```python
from build123d import *
from OCP.BRepFilletAPI import BRepFilletAPI_MakeChamfer

# Parameters (mm, degrees)
SKETCH3_W           = 45.6
SKETCH3_H           = 24.8
BOSS_EXTRUDE1_DEPTH = 29
SKETCH4_W           = 29
SKETCH4_H           = 24.8
BOSS_EXTRUDE2_DEPTH = 1.5
SKETCH6_R           = 12
CUT_EXTRUDE1_DEPTH  = 1.5
BOSS_EXTRUDE3_DEPTH = 1
SKETCH10_W          = 12
SKETCH10_H          = 18.8
BOSS_EXTRUDE5_DEPTH = 1.5
CUT_EXTRUDE2_DEPTH  = 18.8
CUT_EXTRUDE3_DEPTH  = 1.5
SKETCH13_W          = 6
SKETCH13_H          = 20
CUT_EXTRUDE4_DEPTH  = 5
SKETCH14_R          = 0.75
CUT_EXTRUDE5_DEPTH  = 5
SKETCH8_R           = 1
CUT_EXTRUDE6_DEPTH  = 5
CUT_EXTRUDE7_START  = -5
SKETCH15_R          = 0.75
CUT_EXTRUDE7_DEPTH  = 5
SKETCH17_R          = 0.75
CUT_EXTRUDE8_DEPTH  = 5
SKETCH18_R          = 3
BOSS_EXTRUDE6_DEPTH = 3
SKETCH19_R          = 1.5
CUT_EXTRUDE9_DEPTH  = 3
FILLET1_R           = 2
CHAMFER1_SIZE       = 2
CHAMFER2_SIZE       = 1
CHAMFER2_SIZE_2     = 0.577350269
BOSS_EXTRUDE7_START = 3
SKETCH9_R           = 3
SKETCH9_R_2         = 1.25
BOSS_EXTRUDE7_DEPTH = 3


with BuildPart() as part:
    # Sketch3 → Boss-Extrude1 (new body)
    with BuildSketch(Plane(origin=(0, 0, 0), x_dir=(0, 0, -1), z_dir=(1, 0, 0))):
        Rectangle(SKETCH3_W, SKETCH3_H)
    extrude(amount=BOSS_EXTRUDE1_DEPTH)

    # Sketch4 → Boss-Extrude2 (add)
    with BuildSketch(Plane(origin=(29, 0, 0), x_dir=(0, 0, -1), z_dir=(1, 0, 0))):
        with Locations((-8.3, 0)):
            Rectangle(SKETCH4_W, SKETCH4_H)
    boss_extrude2 = extrude(amount=BOSS_EXTRUDE2_DEPTH)

    # Sketch6 → Cut-Extrude1 (cut)
    with BuildSketch(Plane(origin=(29, 0, 0), x_dir=(0, 0, -1), z_dir=(1, 0, 0))):
        with Locations((12.8, 0)):
            Circle(SKETCH6_R)
    cut_extrude1 = extrude(amount=CUT_EXTRUDE1_DEPTH, mode=Mode.SUBTRACT)

    # Sketch7 → Boss-Extrude3 (add)
    with BuildSketch(Plane(origin=(30.5, 0, 0), x_dir=(0, 0, -1), z_dir=(1, 0, 0))):
        with BuildLine():
            Line((-22.8, 7.4), (3.353307457, 7.4))
            ThreePointArc((3.353307457, 7.4), (0.8, 0), (3.353307457, -7.4))
            Line((3.353307457, -7.4), (-22.8, -7.4))
            Line((-22.8, -7.4), (-22.8, 7.4))
        make_face()
    extrude(amount=BOSS_EXTRUDE3_DEPTH)

    # Mirror2: Boss-Extrude2, Cut-Extrude1 across plane
    add(boss_extrude2.mirror(Plane.ZY.offset(-14.5)))
    add(cut_extrude1.mirror(Plane.ZY.offset(-14.5)), mode=Mode.SUBTRACT)

    # Sketch10 → Boss-Extrude5 (add)
    with BuildSketch(Plane.ZY.offset(1.5)):
        with Locations((11.3, 0)):
            Rectangle(SKETCH10_W, SKETCH10_H)
    extrude(amount=BOSS_EXTRUDE5_DEPTH)

    # Sketch11 → Cut-Extrude2 (cut)
    with BuildSketch(Plane.XZ.offset(9.4)):
        Polygon((-3, 7.3), (-1.5, 5.3), (-3, 5.3), align=None)
    extrude(amount=-CUT_EXTRUDE2_DEPTH, mode=Mode.SUBTRACT)

    # Sketch12 → Cut-Extrude3 (cut)
    with BuildSketch(Plane.ZY.offset(1.5)):
        with BuildLine():
            Line((5.3, -10.4), (-0.7, -10.4))
            Line((-0.7, -10.4), (-0.7, -6.479969136))
            Line((-0.7, -6.479969136), (-2.7, -6.479969136))
            ThreePointArc((-2.7, -6.479969136), (-0.8, 0), (-2.7, 6.479969136))
            Line((-2.7, 6.479969136), (-0.7, 6.479969136))
            Line((-0.7, 6.479969136), (-0.7, 9.6))
            Line((-0.7, 9.6), (5.3, 9.6))
            Line((5.3, 9.6), (5.3, -10.4))
        make_face()
    extrude(amount=-CUT_EXTRUDE3_DEPTH, mode=Mode.SUBTRACT)

    # Sketch13 → Cut-Extrude4 (cut)
    with BuildSketch(Plane.ZY):
        with Locations((2.3, -0.4)):
            Rectangle(SKETCH13_W, SKETCH13_H)
    extrude(amount=-CUT_EXTRUDE4_DEPTH, mode=Mode.SUBTRACT)

    # Sketch14 → Cut-Extrude5 (cut)
    with BuildSketch(Plane.ZY.offset(1.5)):
        with Locations((20.8, 10.4)):
            Circle(SKETCH14_R)
        with Locations((20.8, -10.4)):
            Circle(SKETCH14_R)
        with Locations((-3.7, 10.4)):
            Circle(SKETCH14_R)
        with Locations((-3.7, -10.4)):
            Circle(SKETCH14_R)
    extrude(amount=-CUT_EXTRUDE5_DEPTH, mode=Mode.SUBTRACT)

    # Sketch8 → Cut-Extrude6 (cut)
    with BuildSketch(Plane(origin=(30.5, 0, 0), x_dir=(0, 0, -1), z_dir=(1, 0, 0))):
        with Locations((-20.8, 10.4)):
            Circle(SKETCH8_R)
        with Locations((-20.8, -10.4)):
            Circle(SKETCH8_R)
    cut_extrude6 = extrude(amount=-CUT_EXTRUDE6_DEPTH, mode=Mode.SUBTRACT)

    # Sketch15 → Cut-Extrude7 (cut)
    with BuildSketch(Plane(origin=(30.5, 0, 0), x_dir=(0, 0, -1), z_dir=(1, 0, 0)).offset(CUT_EXTRUDE7_START)):
        with Locations(Location((3.7, -10.4, 0), (0, 0, 180))):
            Circle(SKETCH15_R)
        with Locations(Location((3.7, 10.4, 0), (0, 0, 180))):
            Circle(SKETCH15_R)
    extrude(amount=CUT_EXTRUDE7_DEPTH, mode=Mode.SUBTRACT)

    # Sketch17 → Cut-Extrude8 (cut)
    with BuildSketch(Plane(origin=(30.5, 0, 0), x_dir=(0, 0, -1), z_dir=(1, 0, 0))):
        with Locations((-16.8, 10.4)):
            Circle(SKETCH17_R)
        with Locations((-16.8, -10.4)):
            Circle(SKETCH17_R)
    extrude(amount=-CUT_EXTRUDE8_DEPTH, mode=Mode.SUBTRACT)

    # Mirror3: Cut-Extrude6 across plane
    add(cut_extrude6.mirror(Plane.XY), mode=Mode.SUBTRACT)

    # Sketch18 → Boss-Extrude6 (add)
    with BuildSketch(Plane(origin=(29, 0, 0), x_dir=(0, 0, -1), z_dir=(1, 0, 0))):
        with Locations(Location((12.8, 0, 0), (0, 0, 180))):
            Circle(SKETCH18_R)
    extrude(amount=BOSS_EXTRUDE6_DEPTH)

    # Sketch19 → Cut-Extrude9 (cut)
    with BuildSketch(Plane(origin=(32, 0, 0), x_dir=(0, 0, -1), z_dir=(1, 0, 0))):
        with Locations((12.8, 0)):
            Circle(SKETCH19_R)
    extrude(amount=-CUT_EXTRUDE9_DEPTH, mode=Mode.SUBTRACT)

    # Fillet1
    fillet1_edges = [part.edges().sort_by_distance(p)[0] for p in [
        (14.5, -12.4, 22.8),
        (14.5, 12.4, 22.8),
    ]]
    fillet(fillet1_edges, radius=FILLET1_R)

    # Chamfer1
    chamfer1_edges = [part.edges().sort_by_distance(p)[0] for p in [
        (14.5, -12.4, -22.8),
        (14.5, 12.4, -22.8),
    ]]
    chamfer(chamfer1_edges, length=CHAMFER1_SIZE)

    # Chamfer2
    chamfer2_edges_1 = [part.edges().sort_by_distance(p)[0] for p in [
        (30.5, -12.4, 7.3),
    ]]
    chamfer2_side_1 = [part.faces().sort_by_distance(p)[0] for p in [
        (30.488452995, -12.4, 7.3),
    ]]
    chamfer2_edges_2 = [part.edges().sort_by_distance(p)[0] for p in [
        (30.5, 8.9, 22.8),
    ]]
    chamfer2_side_2 = [part.faces().sort_by_distance(p)[0] for p in [
        (30.488452995, 8.9, 22.8),
    ]]
    chamfer2_edges_3 = [part.edges().sort_by_distance(p)[0] for p in [
        (30.5, 12.4, 7.3),
    ]]
    chamfer2_side_3 = [part.faces().sort_by_distance(p)[0] for p in [
        (30.488452995, 12.4, 7.3),
    ]]
    chamfer2_edges_4 = [part.edges().sort_by_distance(p)[0] for p in [
        (30.5, 11.814213562, 22.214213562),
    ]]
    chamfer2_side_4 = [part.faces().sort_by_distance(p)[0] for p in [
        (30.488452995, 11.814213562, 22.214213562),
    ]]
    chamfer2_edges_5 = [part.edges().sort_by_distance(p)[0] for p in [
        (30.5, -11.814213562, 22.214213562),
    ]]
    chamfer2_side_5 = [part.faces().sort_by_distance(p)[0] for p in [
        (30.5, -11.806048597, 22.206048597),
    ]]
    chamfer2_edges_6 = [part.edges().sort_by_distance(p)[0] for p in [
        (30.5, -8.9, 22.8),
    ]]
    chamfer2_side_6 = [part.faces().sort_by_distance(p)[0] for p in [
        (30.5, -8.9, 22.788452995),
    ]]
    chamfer2 = BRepFilletAPI_MakeChamfer(part.part.solid().wrapped)
    for e in chamfer2_edges_1:
        chamfer2.Add(CHAMFER2_SIZE - 0.0001, CHAMFER2_SIZE_2 - 0.0001, e.wrapped, chamfer2_side_1[0].wrapped)
    for e in chamfer2_edges_2:
        chamfer2.Add(CHAMFER2_SIZE_2 - 0.0001, CHAMFER2_SIZE - 0.0001, e.wrapped, chamfer2_side_2[0].wrapped)
    for e in chamfer2_edges_3:
        chamfer2.Add(CHAMFER2_SIZE_2 - 0.0001, CHAMFER2_SIZE - 0.0001, e.wrapped, chamfer2_side_3[0].wrapped)
    for e in chamfer2_edges_4:
        chamfer2.Add(CHAMFER2_SIZE_2 - 0.0001, CHAMFER2_SIZE - 0.0001, e.wrapped, chamfer2_side_4[0].wrapped)
    for e in chamfer2_edges_5:
        chamfer2.Add(CHAMFER2_SIZE_2 - 0.0001, CHAMFER2_SIZE - 0.0001, e.wrapped, chamfer2_side_5[0].wrapped)
    for e in chamfer2_edges_6:
        chamfer2.Add(CHAMFER2_SIZE_2 - 0.0001, CHAMFER2_SIZE - 0.0001, e.wrapped, chamfer2_side_6[0].wrapped)
    add(Compound.cast(chamfer2.Shape()), mode=Mode.REPLACE)  # a hair under: the kernel refuses the full size

    # Sketch9 → Boss-Extrude7 (add)
    with BuildSketch(Plane.ZY.offset(BOSS_EXTRUDE7_START)):
        with Locations((-12.8, 0)):
            Circle(SKETCH9_R)
        with Locations((-12.8, 0)):
            Circle(SKETCH9_R_2, mode=Mode.SUBTRACT)
    extrude(amount=-BOSS_EXTRUDE7_DEPTH)


solid = part.part
```
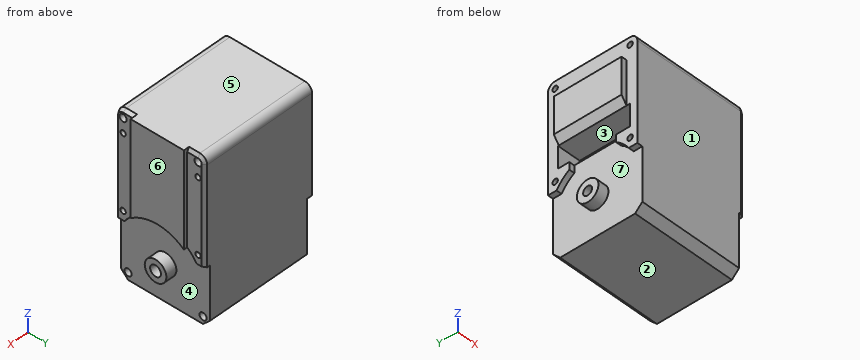
Design review of the part built by this model. Coordinates are the model's own, in mm. Face numbers are marked on the shaded views. A direction names the side the tool comes from. Give positions to 0.01 mm unless a question says otherwise; leave off trailing zeros. Loops run counter-clockwise (first coordinate to the right, second up) from the corner with the lowest first, then second, coordinate; pieces in that order, holes last. Notation, with made-up numbers: (-18.5, 40) -> (40.5, 40) arc R16 ccw to (40.5, 64) -> close; hole circle Ø7 at (81.5, 1.5). An arc over 180 degrees is marked (long way). One line per item, written item: value.
Q1. We need section C-C on z = -5. Give the boundary of the cut face in (x, y), and give its area (3 significant figures).
Numbers:
outline: (-1.5, -12.4) -> (29.5, -12.4) -> (30.5, -11.82) -> (30.5, -9.12) -> (29, -9.12) -> (29, 9.12) -> (30.5, 9.12) -> (30.5, 11.4) -> (29.92, 12.4) -> (-1.5, 12.4) -> (-1.5, 9.12) -> (0, 9.12) -> (0, -9.12) -> (-1.5, -9.12) -> close
area: 738 mm^2
Q2. For pin 1 Ø1.6 at (y, z) = (-10, 20.5) entering from +X; pin 2 Ø4 at (y, z) = (3, -18) entering from +X; pin 3 Ø2.5 at (y, z) = (-10.4, -3.7) entering from -X, all flat-tipped, find the tip position at first contact; note any pin that passes through.
Numbers:
pin 1: stops at x = 30.5
pin 2: stops at x = 29
pin 3: stops at x = -1.5
Q3. For L1, parallel to Y at x = 26.35, z = -20.8; L2, parallel to Y at x = 27, z = 20; L3, parallel to Z at x = 1, y = -4, list the stretches that pass through material, from the lowest coordinate up.
Numbers:
L1: y = -12.4 to -11.4, -9.4 to 9.4, 11.4 to 12.4
L2: y = -12.4 to -11, -9.8 to 9.8, 11 to 12.4
L3: z = -22.8 to -0.7, 5.3 to 22.8
Q4. Machinability: for the marked faces 5, 6 and 7, which of the approach directions +Z, -Z, +X, -X, +Y, -Y give a long, thin tool a straight path to every point of the face, cutting with its end or side? Answer none if there is none.
Numbers:
face 5: +Z, +X, -X, +Y, -Y
face 6: +Z, +X, +Y, -Y
face 7: -X
Q5. Draft analysis for pull direction Z (two halves, no side actions). For the marked faces 1, 2, 3 and 4, state which applies: pulls with the +Z half, pulls with the -Z half, needs draft (parallel to the pull), parting line crosses it, or undercut.
Numbers:
face 1: needs draft
face 2: pulls with the -Z half
face 3: undercut
face 4: undercut
Q6. We need section B-B on z = 4.5. Give the boundary of the cut face in (x, y).
Numbers:
outline: (-1.5, -12.4) -> (29.5, -12.4) -> (30.5, -11.82) -> (30.5, -7.4) -> (31.5, -7.4) -> (31.5, 7.4) -> (30.5, 7.4) -> (30.5, 11.4) -> (29.92, 12.4) -> (-1.5, 12.4) -> (-1.5, 9.6) -> (5, 9.6) -> (5, -10.4) -> (-1.5, -10.4) -> close
